The listing builds one solid part. Answer for the finished solid, in the listing's coordinates (mm). Face numbers are marked on the shaded views. A direction names the side the tool comes from. Give positions to 0.01 mm unless a question says otherwise; leave off trailing zeros. Order: outer loops, then holes, each group sorted by start corner. A loop starts at its lowest first (then second) coordinate and runs counter-clockwise, first axis right, second up. Notation, with made-up numbers: (84.25, 36.5) -> (143.25, 36.5) arc R22 cw to (143.25, 53.5) -> close; hole circle Ø2 at (-6, 17.25). An arc over 180 degrees is marked (long way). Write item = value, one per line. Start each with the question number.
```python
from build123d import *

# Parameters (mm, degrees)
SKETCH_1_W           = 34
SKETCH_1_H           = 30
EXTRUDE_1_DEPTH      = 22
EXTRUDE_1_2_DEPTH    = 22
EXTRUDE_2_DEPTH      = 4.5
EXTRUDE_2_DEPTH_BACK = 75
SKETCH_2_R           = 3.5
SKETCH_3_R           = 2.05
CUT_EXTRUDE_1_DEPTH  = 5


with BuildPart() as part:
    # Sketch 1 → Extrude 1 (new body)
    with BuildSketch(Plane(origin=(0, 0, 0), x_dir=(1, 0, 0), z_dir=(0, 1, 0))):
        Rectangle(SKETCH_1_W, SKETCH_1_H)
    extrude(amount=EXTRUDE_1_DEPTH)



with BuildPart() as body_2:
    # Sketch 1 → Extrude 1 2 (new body)
    with BuildSketch(Plane(origin=(0, 0, 0), x_dir=(1, 0, 0), z_dir=(0, 1, 0))):
        with Locations((0, 42)):
            Rectangle(SKETCH_1_W, SKETCH_1_H)
    extrude(amount=EXTRUDE_1_2_DEPTH)


with BuildPart() as part_1:
    add(part.part)

    add(body_2.part)  # Extrude 2 merges body 2
    # Sketch 2 → Extrude 2 (add, two sides: drawn at the far end of the back side and taken through both)
    with BuildSketch(Plane.XY.offset(15).offset(-EXTRUDE_2_DEPTH_BACK)):
        with Locations((0, 11)):
            Circle(SKETCH_2_R)
    extrude(amount=EXTRUDE_2_DEPTH + EXTRUDE_2_DEPTH_BACK)

    # Sketch 3 → Cut-Extrude 1 (cut)
    with BuildSketch(Plane(origin=(0, 0, 0), x_dir=(-1, 0, 0), z_dir=(0, -1, 0))):
        with Locations(Location((-11.75, 33.25, 0), (0, 0, 90))):
            Circle(SKETCH_3_R)
        with Locations(Location((11.75, 33.25, 0), (0, 0, 90))):
            Circle(SKETCH_3_R)
        with Locations(Location((11.75, 50.75, 0), (0, 0, 90))):
            Circle(SKETCH_3_R)
        with Locations(Location((-11.75, 50.75, 0), (0, 0, 90))):
            Circle(SKETCH_3_R)
        with Locations(Location((-12, -9, 0), (0, 0, 90))):
            Circle(SKETCH_3_R)
        with Locations(Location((-12, 9, 0), (0, 0, 90))):
            Circle(SKETCH_3_R)
        with Locations(Location((12, 9, 0), (0, 0, 90))):
            Circle(SKETCH_3_R)
        with Locations(Location((12, -9, 0), (0, 0, 90))):
            Circle(SKETCH_3_R)
    extrude(amount=-CUT_EXTRUDE_1_DEPTH, mode=Mode.SUBTRACT)


solid = part_1.part
```
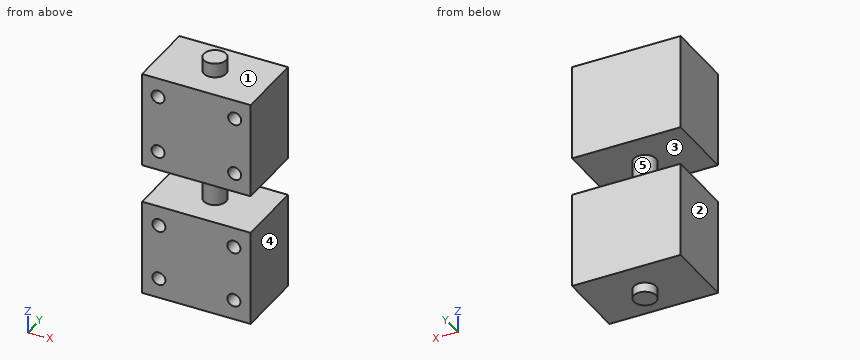
Item 1: A cutting plane is placed at C-C, the plane x = 0. Write down the section's boundary in (y, z).
Item 2: Flat-ended cylindrical pins translate along their axes: pin 1 (1.5 mm diameter, centred on x = 12.5, y = 3, fed in from -Z); pin 2 (1 mm diameter, centred on x = 1, z = -23.5, fed in from +Y); pin 3 (1.2 mm diameter, centred on x = 12, z = -32.5, fed in from -Y). Find the tip coordinate at first contact, or state that the pin passes through.
Item 3: A cutting plane is placed at D-D, the plane y = 11. Write down the section's boundary in (x, z), plus the area to 3 significant figures.
Item 4: Consider L1, parallel to X at y = 1.9, z = -9; L2, parallel to X at y = 1.8, z = -50.75; L3, parallel to Z at x = -7.5, y = 21.25. Determine where each line is inside the solid, lowest interval first. Write a range as from..to.
Item 5: A cutting plane is placed at A-A, the plane x = -7.5. Write down the section's boundary in (y, z), plus the area to 3 significant figures.
Item 6: Which of the six approach directions +Z, -Z, +X, -X, +Y, -Y give full straight-line access (tool end or side, diameter ignored) to the marked faces 4 and 5?
Item 7: The mould has two halves that part along Z. Classify the marked faces 1, 2 and 3: +Z half, -Z half, draft (parallel to the pull), parting line (faces both ways), or undercut.
Item 8: A cutting plane is placed at B-B, the plane z = 9. Write down the section's boundary in (x, y).
Check values:
q1.outline = (0, -57) -> (7.5, -57) -> (7.5, -60) -> (14.5, -60) -> (14.5, -57) -> (22, -57) -> (22, -27) -> (14.5, -27) -> (14.5, -15) -> (22, -15) -> (22, 15) -> (14.5, 15) -> (14.5, 19.5) -> (7.5, 19.5) -> (7.5, 15) -> (0, 15) -> (0, -15) -> (7.5, -15) -> (7.5, -27) -> (0, -27) -> close
q2.pin_1 = -57
q2.pin_2 = 14.46
q2.pin_3 = 5
q3.outline = (-17, -57) -> (-3.5, -57) -> (-3.5, -60) -> (3.5, -60) -> (3.5, -57) -> (17, -57) -> (17, -27) -> (3.5, -27) -> (3.5, -15) -> (17, -15) -> (17, 15) -> (3.5, 15) -> (3.5, 19.5) -> (-3.5, 19.5) -> (-3.5, 15) -> (-17, 15) -> (-17, -15) -> (-3.5, -15) -> (-3.5, -27) -> (-17, -27) -> close
q3.area = 2,180 mm^2
q4.L1 = -17..-14.05, -9.95..9.95, 14.05..17
q4.L2 = -17..-13.8, -9.7..9.7, 13.8..17
q4.L3 = -57..-27, -15..15
q5.outline = (0, -57) -> (22, -57) -> (22, -27) -> (0, -27) -> close; (0, -15) -> (22, -15) -> (22, 15) -> (0, 15) -> close
q5.area = 1,320 mm^2
q6.face_4 = +Z, -Z, +X, +Y, -Y
q6.face_5 = none
q7.face_1 = +Z half
q7.face_2 = draft
q7.face_3 = undercut
q8.outline = (-17, 0) -> (-14.05, 0) -> (-14.05, 5) -> (-9.95, 5) -> (-9.95, 0) -> (9.95, 0) -> (9.95, 5) -> (14.05, 5) -> (14.05, 0) -> (17, 0) -> (17, 22) -> (-17, 22) -> close
